Input: part model. Units: mm. Frame: model coordinates. A direction names the side the tool comes from. Coordinates: 2 decimals unless noted, no trailing zeros. Order: outer loops, then holes, each group sorted by start corner. A loop starts at its lowest first (then second) coordinate and runs counter-clockwise, first axis right, second up.
Autodesk Fusion 360 part; units mm, degrees
sketch "Esquisse1" plane through (0, 0, 0) normal (1, 0, 0) x (0, 1, 0)
  line L0 (0, 0) -> (-16, 0)
  line L1 (-16, 0) -> (-16, 6.5037)
  line L2 (-16, 6.5037) -> (-15.2163, 6.5037)
  line L3 (-15.2163, 6.5037) -> (-15.2163, 9.9566)
  line L4 (-15.2163, 9.9566) -> (-11.3366, 9.9566)
  line L5 (-11.3366, 9.9566) -> (-11.3366, 23)
  line L6 (-11.3366, 23) -> (0, 23)
  line L7 (0, 23) -> (0, 0)
  line L8 (0, 2.5) -> (0, 20)
  dimension "d1" = 16
  dimension "d2" = 15.2163
revolve "Révolution1" add sketch "Esquisse1" angle 360 about axis through (0, 0, 23) along (0, 0, -1)
Item 1: Ray query, probe 1 along X at (y, z) = (0.5, 9.25); probe 2 along Z at (x, y) = (12, 2); probe 3 along Z at (x, y) = (11.5, 10.5). Return the intervals inside material, ascending.
Response values:
probe 1: x = -15.21 to 15.21
probe 2: z = 0 to 9.96
probe 3: z = 0 to 6.5
Item 2: Access query for faces 1 (the face through (0, 0, 0)), 2 (the face through (3.41, -10.81, 16.57)). Directions: +Z, -Z, +X, -X, +Y, -Y. A direction counts if a zero-diameter tool reaches every point of the face in a straight line with its end or side. Return the directions, or none.
Response values:
face 1: -Z, +X, -X, +Y, -Y
face 2: +Z
Item 3: Cut plane D-D on z = 8. Return loops of the section in (x, y).
Response values:
outline: circle Ø30.43 at (0, 0)
Item 4: Cut plane A-A on y = 0. Return loops of the section in (x, z), then the cut area to 3 significant figures.
Response values:
outline: (-16, 0) - (16, 0) - (16, 6.5) - (15.22, 6.5) - (15.22, 9.96) - (11.34, 9.96) - (11.34, 23) - (-11.34, 23) - (-11.34, 9.96) - (-15.22, 9.96) - (-15.22, 6.5) - (-16, 6.5) - close
area: 609 mm2
Item 5: Pin query (flat end, axial travel): pin 1 Ø2 at (y, z) = (11, 7) entering from -X; pin 2 Ø4 at (x, z) = (5.5, 16.5) entering from +Y; pin 3 Ø8 at (x, z) = (4, 9) entering from +Y. Return the tip coordinate at first contact, or that it passes through.
Response values:
pin 1: stops at x = -12.38
pin 2: stops at y = 10.78
pin 3: stops at y = 15.98
Item 6: Cut plane B-B on z = 21.5. Return loops of the section in (x, y).
Response values:
outline: circle Ø22.67 at (0, 0)
Item 7: Cut plane C-C on x = 3.5. Return loops of the section in (y, z).
Response values:
outline: (-15.61, 0) - (15.61, 0) - (15.61, 6.5) - (14.81, 6.5) - (14.81, 9.96) - (10.78, 9.96) - (10.78, 23) - (-10.78, 23) - (-10.78, 9.96) - (-14.81, 9.96) - (-14.81, 6.5) - (-15.61, 6.5) - close
